For this review, use the dimensioned drawing (mm, ordinates from the lowest corner) and the shaded views. A direction names the side the tool comes from. Coordinates: 2 decimals unless noted, no trailing zeros. Loops run counter-clockwise (first coordinate to the right, second up) from the corner with the lowest first, then second, coordinate; pieces in that order, holes last. Notation, with made-up numbers: (29.5, 44) - (62.5, 44) arc R17 ccw to (62.5, 50) - close; hole circle Ø7 at (-29.5, 85). An arc over 180 degrees is marked (long way). Answer in a Markdown table with one row per item. Add a question column.
(1) We need section B-B, the plane z = 30. Write out the cut boundary in (x, y), plus the area to 3 significant figures.
(2) Clearance check with flat-ended pins moving along their axes: pin 1 (2 mm diameter, centred on x = 17, y = 22, fed in from -Z); pin 2 (8 mm diameter, centred on x = 24, y = 21.5, fed in from -Z); pin 3 (4 mm diameter, centred on x = 29.5, y = 28, fed in from +Z). State where each tip first meets the part, or that it passes through.
(3) The part is to be moulded in two halves that separate along X. For the marked faces 3, 4 and 5, say which applies: released by +X, released by -X, zero draft, split by the parting line, or undercut.
(4) To check wall thickness, follow L1, parallel to Z at x = 30, y = 31.5; L2, parallel to Z at x = 30, y = 33.5. State the ranges of each line that lie inside material, in increasing order. Write a range as [from, to].
(5) For the marked faces 1 and 2, list the 3-axis set-ups (+Z, -Z, +X, -X, +Y, -Y) from which the entire face can be reached by the end or side of a thin tool; tool diameter is ignored.
(6) We need section A-A, the plane x = 30. Write out the cut boundary in (y, z).
(7) We need section C-C, the plane y = 20. Write out the cut boundary in (x, z), plus the area to 3 significant figures.
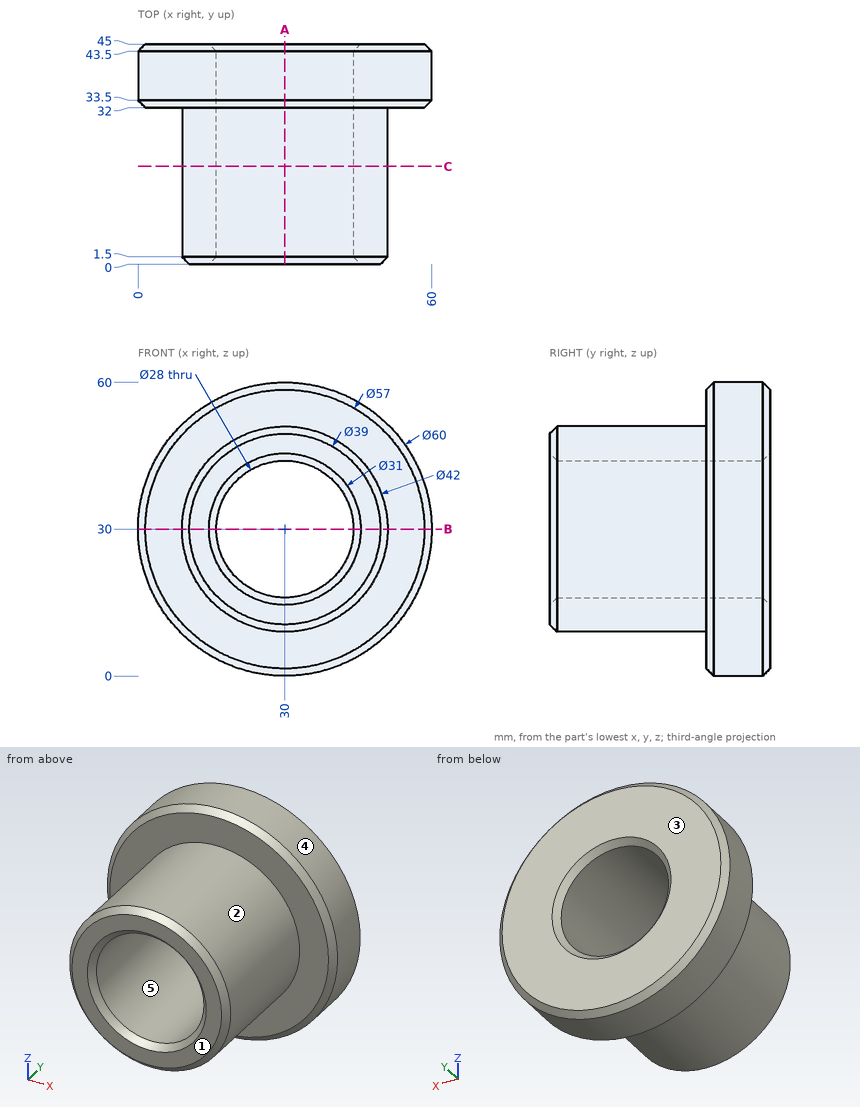
Responses:
| question | item | result |
|---|---|---|
| 1 | outline | (0, 33.5) - (1.5, 32) - (9, 32) - (9, 1.5) - (10.5, 0) - (14.5, 0) - (16, 1.5) - (16, 43.5) - (14.5, 45) - (1.5, 45) - (0, 43.5) - close; (44, 1.5) - (45.5, 0) - (49.5, 0) - (51, 1.5) - (51, 32) - (58.5, 32) - (60, 33.5) - (60, 43.5) - (58.5, 45) - (45.5, 45) - (44, 43.5) - close |
| 1 | area | 853 mm2 |
| 2 | pin 1 | stops at z = 12.77 |
| 2 | pin 2 | stops at z = 9.1 |
| 2 | pin 3 | stops at z = 51 |
| 3 | face 3 | zero draft |
| 3 | face 4 | split by the parting line |
| 3 | face 5 | undercut |
| 4 | L1 | z = [9, 16], [44, 51] |
| 4 | L2 | z = [0, 16], [44, 60] |
| 5 | face 1 | +Z, -Z, +X, -X, -Y |
| 5 | face 2 | -Y |
| 6 | outline | (0, 10.5) - (1.5, 9) - (32, 9) - (32, 1.5) - (33.5, 0) - (43.5, 0) - (45, 1.5) - (45, 14.5) - (43.5, 16) - (1.5, 16) - (0, 14.5) - close; (0, 45.5) - (1.5, 44) - (43.5, 44) - (45, 45.5) - (45, 58.5) - (43.5, 60) - (33.5, 60) - (32, 58.5) - (32, 51) - (1.5, 51) - (0, 49.5) - close |
| 7 | outline | circle Ø42 at (30, 30); hole circle Ø28 at (30, 30) |
| 7 | area | 770 mm2 |
